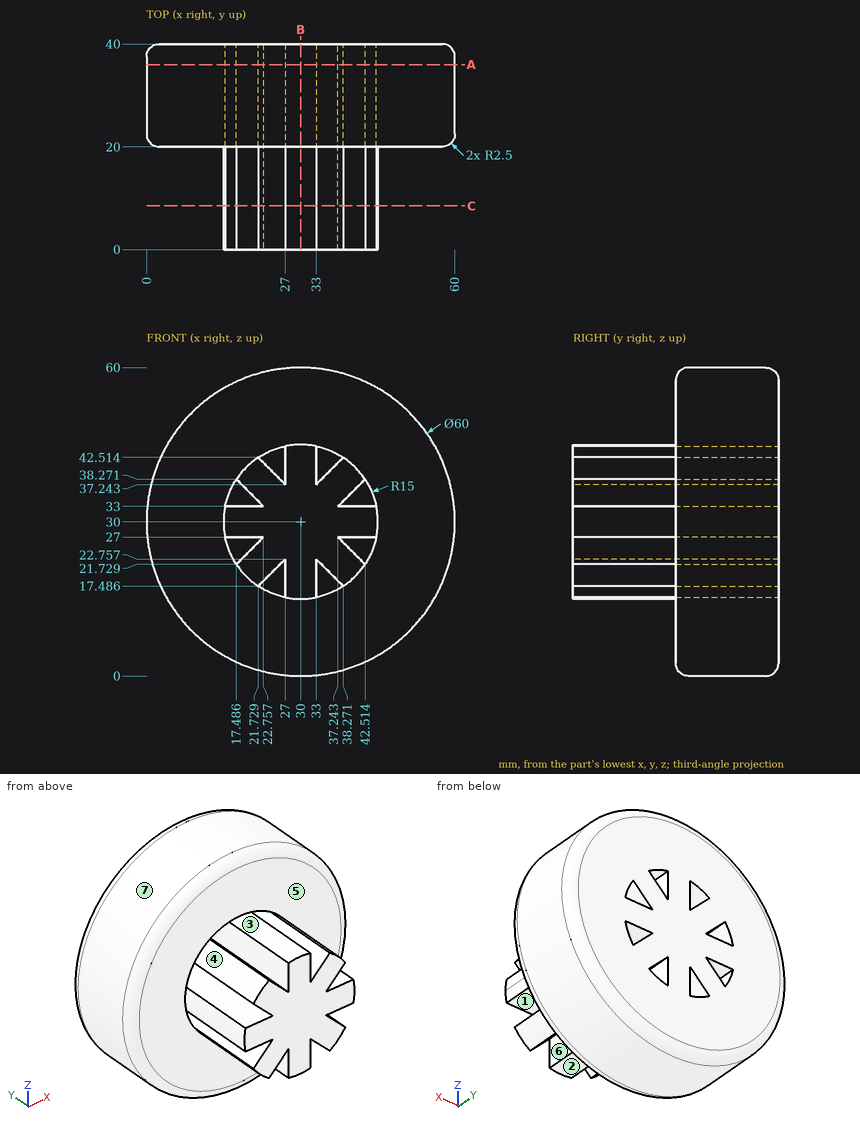
Part print with two shaded views. Sizes in mm from the minimum x, y, z corner. A direction names the side the tool comes from. Coordinates: 2 decimals unless noted, no trailing zeros. Write each loop counter-clockwise with the first axis right and the second up, starting at its lowest first coordinate (ties: lowest second). Pieces come first, ordered by that corner, then holes.
(1) Cut at B-B on x = 30. List the corners of the cut face in (y, z).
(2) 3-axis set-ups, long thin cutter, end or side, ignore diameter. For the marked faces 1, 2, 3 and 4: which of +Z, -Z, +X, -X, +Y, -Y reach the whole face in a straight line?
(3) Drill centre lines: line 1 (X direction, y = 30, z = 38) (1 decimal); line 2 (Z direction, x = 16.5, y = 23) (1 decimal); line 3 (Z direction, x = 19, y = 4) (1 decimal). Where is each one in solid material? Low to high.
(4) Cut at C-C on y = 8.5. List the corners of the cut face in (x, z).
(5) Pin check, flat tips, straight feed: pin 1 Ø2 at (y, z) = (16, 18.5) entering from +X; pin 2 Ø5 at (x, y) = (18, 33.5) entering from +Z; pin 3 Ø10 at (x, y) = (34, 29) entering from +Z. Stop position of each tip, or through.
(6) Mould opens along X. For the marked faces 5, 6 and 7 say: pulls with the +X half, pulls with the -X half, needs draft (parallel to the pull), parting line crosses it, or undercut.
(7) Cut at A-A on y = 36. State how many separate pieces and enclosed holes the cut face has, and give its area (3 significant figures).
Working result:
1. outline: (0, 15) - (20, 15) - (20, 2.5) arc R2.5 ccw to (22.5, 0) - (37.5, 0) arc R2.5 ccw to (40, 2.5) - (40, 57.5) arc R2.5 ccw to (37.5, 60) - (22.5, 60) arc R2.5 ccw to (20, 57.5) - (20, 45) - (0, 45) - close
2. face 1: +Y, -Y
2. face 2: -Z, -Y
2. face 3: +Z, -Y
2. face 4: +Z, -X, -Y
3. line 1: x = 1.1 to 17.3, 17.8 to 26.2, 27 to 33, 33.8 to 42.2, 42.7 to 58.9
3. line 2: z = 3.2 to 23.5, 27 to 33, 36.5 to 56.8
3. line 3: z = 19.8 to 23.2, 27 to 33, 36.8 to 40.2
4. outline: (15.3, 27) - (22.76, 27) - (17.49, 21.73) arc R15 ccw to (21.73, 17.49) - (27, 22.76) - (27, 15.3) arc R15 ccw to (33, 15.3) - (33, 22.76) - (38.27, 17.49) arc R15 ccw to (42.51, 21.73) - (37.24, 27) - (44.7, 27) arc R15 ccw to (44.7, 33) - (37.24, 33) - (42.51, 38.27) arc R15 ccw to (38.27, 42.51) - (33, 37.24) - (33, 44.7) arc R15 ccw to (27, 44.7) - (27, 37.24) - (21.73, 42.51) arc R15 ccw to (17.49, 38.27) - (22.76, 33) - (15.3, 33) arc R15 ccw to start
5. pin 1: stops at x = 40.71
5. pin 2: stops at z = 58.46
5. pin 3: stops at z = 60
6. face 5: needs draft
6. face 6: undercut
6. face 7: parting line crosses it
7. separate pieces: 1
7. enclosed holes: 8
7. area: 2,660 mm2
